```python
from build123d import *

# Parameters (mm, degrees)
F1_DEPTH = 25.4
F3_W     = 9.144
F3_H     = 7.112
F4_DEPTH = 6.3936169982
F5_DEPTH = 6.35
F6_SIZE2 = 2.54
F6_SIZE  = 5.08


with BuildPart() as f1:
    # F0 (on Front) → F1 (new body)
    with BuildSketch(Plane.XZ):
        Polygon((82.1067863703, 44.9580137503), (75.7567863703, 44.9580137503), (75.7567863703, 34.2138137503), (69.3631693721, 34.2138137503), (69.3631693721, 27.1018137503), (75.7567863703, 27.1018137503), (75.7567863703, -46.4819862497), (82.1067863703, -46.4819862497), align=None)
    extrude(amount=F1_DEPTH)

    # F3 (on face) → F4 (cut, through all)
    with BuildSketch(Plane(origin=(69.3631693721, 0, 0), x_dir=(0, -1, 0), z_dir=(-1, 0, 0))):
        with Locations((12.7, 30.6578137503)):
            Rectangle(F3_W, F3_H)
    extrude(amount=-F4_DEPTH, mode=Mode.SUBTRACT)

    # F2 (on face) → F5 (cut, through all)
    with BuildSketch(Plane.YZ.offset(82.1067863703)):
        with BuildLine():
            ThreePointArc((-9.525, 30.3022137503), (-10.4549359697, 32.5472777806), (-12.7, 33.4772137503))
            ThreePointArc((-12.7, 33.4772137503), (-14.9450640303, 28.05714972), (-9.525, 30.3022137503))
        make_face()
    extrude(amount=-F5_DEPTH, mode=Mode.SUBTRACT)

    # F6
    f6_edges = [f1.edges().sort_by_distance(p)[0] for p in [
        (78.931786, -25.4, -46.481986),
        (78.931786, 0, -46.481986),
    ]]
    f6_side = f1.faces().sort_by_distance((78.931786, -12.7, -46.481986))[0]
    chamfer(f6_edges, length=F6_SIZE, length2=F6_SIZE2, reference=f6_side)


solid = f1.part
```
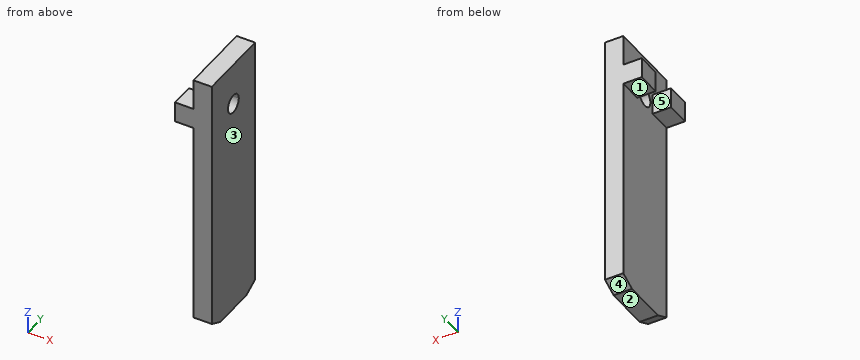
Input: part model. Units: mm. Frame: model coordinates. Face numbers are marked on the shaded views. A direction names the side the tool comes from. Round coordinates to 2 decimals unless told otherwise and drop trailing zeros. Order: outer loops, then holes, each group sorted by start corner. A loop starts at its lowest first (then second) coordinate and runs counter-clockwise, first axis right, second up. Notation, with made-up numbers: (74, 43.25) - (84, 43.25) arc R21 ccw to (84, 52.25) - close; hole circle Ø6 at (-34, 27). An arc over 180 degrees is marked (long way). One line per question, with ' | ' between items. Start each with the question number.
1) Pull-direction query (Y, two-part tool) for the marked faces 3, 4 and 5; classes: +Y half, -Y half, draft (parallel to the pull), parting line (faces both ways), or undercut.
2) Set-up query: the marked faces 1 and 2. Return all of +Z, -Z, +X, -X, +Y, -Y with unobstructed straight access to the full face (end or side cutting, diameter ignored); none if empty.
3) Ray query, probe 1 along Z at (x, y) = (77.5, -12.7); probe 2 along Y at (x, z) = (73, 31.5); probe 3 along X at (y, z) = (-21.5, -28). Return the intervals inside material, ascending.
4) Cut plane D-D, the plane z = -1.5. Return the cut outline in (x, y).
5) Cut plane C-C, the plane y = -21.75. Return the cut outline in (x, z), then the cut area to 3 significant figures.
6) Contact query for flat-ended pins moving along their axis: P1, Ø5, axis at x = 72, y = -23, coming from the +Z side; P2, Ø3, axis at x = 73.5, y = -21.5, coming from the -Z side; P3, Ø6, axis at x = 72.5, y = -14, coming from the +Z side. Output: stop coordinate, or through.
7) Cut plane B-B, the plane x = 73.5. Return the cut outline in (y, z).
8) Cut plane A-A, the plane x = 77.5. Return the cut outline in (y, z) (3 decimals).
Worked out:
1) face 3: draft | face 4: +Y half | face 5: undercut
2) face 1: -Z, -X, +Y, -Y | face 2: -Z, +X, -X, +Y, -Y
3) probe 1: z = -46.48 to 27.13, 33.48 to 44.96 | probe 2: y = -25.4 to -17.27, -8.13 to 0 | probe 3: x = 75.76 to 82.11
4) outline: (75.76, -25.4) - (82.11, -25.4) - (82.11, 0) - (75.76, 0) - close
5) outline: (69.36, 27.1) - (75.76, 27.1) - (75.76, -45.77) - (82.11, -45.77) - (82.11, 44.96) - (75.76, 44.96) - (75.76, 34.21) - (69.36, 34.21) - close | area: 622 mm^2
6) P1: stops at z = 34.21 | P2: stops at z = 27.1 | P3: passes through
7) outline: (-25.4, 27.1) - (-17.27, 27.1) - (-17.27, 34.21) - (-25.4, 34.21) - close; (-8.13, 27.1) - (0, 27.1) - (0, 34.21) - (-8.13, 34.21) - close
8) outline: (-25.4, -43.942) - (-20.32, -46.482) - (-5.08, -46.482) - (0, -43.942) - (0, 44.958) - (-25.4, 44.958) - close; hole circle Ø6.35 at (-12.7, 30.302)
